Can you work these out from the model? Positions are in its coordinate system, mm. A direction names the side the tool comes from. Round coordinates to 2 decimals unless told otherwise and drop trailing zeros. Loops run counter-clockwise (first coordinate to the right, second up) from the corner with the lowest first, then second, coordinate; pieces in that order, holes last.
(1) I want a section at B-B on x = 0. Write out the boundary of the cut face in (y, z).
(2) I want a section at C-C on z = 20. Write out the boundary of the cut face in (x, y), plus the area to 3 significant figures.
(3) Will these pins go through, and if not, where does the flat tip stop? pin 1 Ø1.5 at (x, y) = (4, 55.5) entering from +Z; pin 2 Ø8 at (x, z) = (3.5, 33.5) entering from +Y; pin 3 Ø10.5 at (x, z) = (-1, -0.5) entering from +Y; pin 4 Ø6 at (y, z) = (65, -2.5) entering from +X.
(4) If I drill on line 1 along Y through (x, z) = (0.25, 27.5); line 2 along Z through (x, y) = (-9, 34); line 3 along Z through (x, y) = (2, 65), over which ranges is the centre line in solid material (lowest first)?
(5) Which directions (+Z, -Z, +X, -X, +Y, -Y) give clear straight access to the entire face, cutting with the end or side of a thin tool? Please do faces 4 (the face through (1.3, 63.905, -0.944)), 5 (the face through (0, 7, -4)), 6 (the face through (0.651, 74.717, 30.213)), 7 (the face through (0, 70, 51)), 8 (the face through (0, 3, -10)).
(6) I want a section at A-A on y = 69.76. Write out the boundary of the cut face in (x, z), plus the area to 3 significant figures.
(7) I want a section at D-D on x = -7.5. Write out the boundary of the cut face in (y, z).
(8) Thinking about a two-plate mould opening in Y: for faces 1 (the face through (0, 70, -5)), 2 (the face through (0, 43, 3)), 3 (the face through (0, 78.96, 6)), which applies, released by +Y, released by -Y, zero draft, split by the parting line, or undercut?
from build123d import *

# Parameters (mm, degrees)
SKETCH_2_W      = 20
SKETCH_2_H      = 20
EXTRUDE_2_DEPTH = 7
SKETCH_4_W      = 20
SKETCH_4_H      = 7
EXTRUDE_3_DEPTH = 78.96
SKETCH_5_R      = 5
EXTRUDE_4_DEPTH = 48
SKETCH_10_R     = 5.997428606
EXTRUDE_5_DEPTH = 8


with BuildPart() as part:
    # Эскиз2 → Бобышка-Вытянуть2 (new body)
    with BuildSketch(Plane(origin=(0, 0, 0), x_dir=(1, 0, 0), z_dir=(0, 1, 0))):
        Rectangle(SKETCH_2_W, SKETCH_2_H)
    extrude(amount=EXTRUDE_2_DEPTH)

    # Эскиз4 → Бобышка-Вытянуть3 (add)
    with BuildSketch(Plane(origin=(0, 0, 0), x_dir=(-1, 0, 0), z_dir=(0, -1, 0))):
        with Locations((0, -6.5)):
            Rectangle(SKETCH_4_W, SKETCH_4_H)
    extrude(amount=-EXTRUDE_3_DEPTH)

    # Эскиз5 → Бобышка-Вытянуть4 (add)
    with BuildSketch(Plane(origin=(0, 0, 3), x_dir=(-1, 0, 0), z_dir=(0, 0, -1))):
        with Locations((0, 69.76)):
            Circle(SKETCH_5_R)
    extrude(amount=-EXTRUDE_4_DEPTH)

    # Эскиз10 → Бобышка-Вытянуть5 (add)
    with BuildSketch(Plane(origin=(0, 0, 3), x_dir=(-1, 0, 0), z_dir=(0, 0, -1))):
        with Locations((0, 69.76)):
            Circle(SKETCH_10_R)
    extrude(amount=EXTRUDE_5_DEPTH)


solid = part.part
Filled sheet:
1. outline: (0, -10) - (7, -10) - (7, 3) - (63.76, 3) - (63.76, -5) - (75.76, -5) - (75.76, 3) - (78.96, 3) - (78.96, 10) - (74.76, 10) - (74.76, 51) - (64.76, 51) - (64.76, 10) - (0, 10) - close
2. outline: circle Ø10 at (0, 69.76)
2. area: 78.5 mm2
3. pin 1: stops at z = 10
3. pin 2: stops at y = 74.76
3. pin 3: stops at y = 78.96
3. pin 4: stops at x = 5.73
4. line 1: y = 64.77 to 74.75
4. line 2: z = 3 to 10
4. line 3: z = -5 to 10
5. face 4: -Z
5. face 5: -Z, +X, -X
5. face 6: +Z
5. face 7: +Z, +X, -X, +Y, -Y
5. face 8: -Z, +X, -X, +Y, -Y
6. outline: (-10, 3) - (-6, 3) - (-6, -5) - (6, -5) - (6, 3) - (10, 3) - (10, 10) - (5, 10) - (5, 51) - (-5, 51) - (-5, 10) - (-10, 10) - close
6. area: 646 mm2
7. outline: (0, -10) - (7, -10) - (7, 3) - (78.96, 3) - (78.96, 10) - (0, 10) - close
8. face 1: zero draft
8. face 2: undercut
8. face 3: released by +Y
